The listing builds one solid part. Answer for the finished solid, in the listing's coordinates (mm). Coordinates: 2 decimals unless noted, no trailing zeros. Loops run counter-clockwise (first coordinate to the right, second up) from the corner with the lowest first, then second, coordinate; pieces in that order, holes last. Notation, with made-up numbers: (-15.5, 62) - (4.5, 62) arc R21 cw to (4.5, 97) - close; hole circle Ø9 at (39, -11). An arc over 180 degrees is marked (long way). Return JSON: item names as keys, results as strings. Group by question number.
1. Section B-B (z = 1.5) is taken. State how many separate pieces and enclosed holes the cut face has, and give its area (3 significant figures).
2. Each of these flat-tipped pins is pushed along its axis until it touches: P1, Ø0.8, axis at x = 399, z = 1.5, coming from the -Y side; P2, Ø0.6, axis at y = 21, z = 1, coming from the -X side. Where does it stop, or does it pass through?
3. Find the intervals of material crossed by line 1 along X through (y, z) = (32, 0.55); line 2 along Y through (x, z) = (221.5, 1.5); line 3 along Y through (x, z) = (230, 0.5), in increasing order.
4. Section A-A (x = 232) is taken. Write down the section's boundary in (y, z).
5. Section C-C (x = 328.5) is taken. Write down the section's boundary in (y, z).
```python
from build123d import *

# Parameters (mm, degrees)
SKETCH_2_W      = 1.5
SKETCH_2_H      = 6
EXTRUDE_2_DEPTH = 2


with BuildPart() as part:
    # 草图2 → 凸台-拉伸2 (new body)
    with BuildSketch(Plane.XY):
        Polygon((8.053783248, 22.194978349), (6.553783248, 22.194978349), (6.553783248, 28.194978349), (8.053783248, 28.194978349), (8.053783248, 34.194978349), (533.429113931, 35.353824286), (533.429113931, 5.627058882), (8.053783248, 16.095153128), align=None)
        with Locations((128.889742021, 24.455033291)):
            Rectangle(SKETCH_2_W, SKETCH_2_H, mode=Mode.SUBTRACT)
        with Locations((258.982626832, 23.318434437)):
            Rectangle(SKETCH_2_W, SKETCH_2_H, mode=Mode.SUBTRACT)
        with Locations((399.123508139, 22.161638966)):
            Rectangle(SKETCH_2_W, SKETCH_2_H, mode=Mode.SUBTRACT)
        with BuildLine():
            Line((14.053783248, 26.212604877), (14.053783248, 23.93734113))
            ThreePointArc((14.053783248, 23.93734113), (14.625552855, 22.537284723), (16.013941191, 21.937738017))
            Line((16.013941191, 21.937738017), (46.013941191, 21.339988544))
            ThreePointArc((46.013941191, 21.339988544), (47.453839655, 21.911361263), (48.053783248, 23.339591657))
            Line((48.053783248, 23.339591657), (48.053783248, 26.278777337))
            ThreePointArc((48.053783248, 26.278777337), (47.466436254, 27.694549736), (46.049371762, 28.278772471))
            Line((46.049371762, 28.278772471), (16.049371762, 28.212600011))
            ThreePointArc((16.049371762, 28.212600011), (14.638010849, 27.625257882), (14.053783248, 26.212604877))
        make_face(mode=Mode.SUBTRACT)
        with BuildLine():
            Line((52.053783248, 26.362790255), (52.053783248, 23.180191797))
            ThreePointArc((52.053783248, 23.180191797), (52.625552855, 21.78013539), (54.013941191, 21.180588684))
            Line((54.013941191, 21.180588684), (82.099899964, 20.620976448))
            ThreePointArc((82.099899964, 20.620976448), (83.539798428, 21.192349168), (84.139742021, 22.620579561))
            Line((84.139742021, 22.620579561), (84.139742021, 26.362790255))
            ThreePointArc((84.139742021, 26.362790255), (83.553955584, 27.777003817), (82.139742021, 28.362790255))
            Line((82.139742021, 28.362790255), (54.053783248, 28.362790255))
            ThreePointArc((54.053783248, 28.362790255), (52.639569686, 27.777003817), (52.053783248, 26.362790255))
        make_face(mode=Mode.SUBTRACT)
        with BuildLine():
            Line((88.139742021, 26.376019882), (88.139742021, 22.461179702))
            ThreePointArc((88.139742021, 22.461179702), (88.711511628, 21.061123295), (90.099899964, 20.461576589))
            Line((90.099899964, 20.461576589), (120.099899964, 19.863827115))
            ThreePointArc((120.099899964, 19.863827115), (121.539798428, 20.435199835), (122.139742021, 21.863430228))
            Line((122.139742021, 21.863430228), (122.139742021, 26.442192342))
            ThreePointArc((122.139742021, 26.442192342), (121.552395026, 27.857964741), (120.135330535, 28.442187476))
            Line((120.135330535, 28.442187476), (90.135330535, 28.376015016))
            ThreePointArc((90.135330535, 28.376015016), (88.723969622, 27.788672887), (88.139742021, 26.376019882))
        make_face(mode=Mode.SUBTRACT)
        with BuildLine():
            Line((135.639742021, 26.480792944), (135.639742021, 21.514743035))
            ThreePointArc((135.639742021, 21.514743035), (136.211511628, 20.114686628), (137.599899964, 19.515139922))
            Line((137.599899964, 19.515139922), (170.499899964, 18.859607999))
            ThreePointArc((170.499899964, 18.859607999), (171.939798428, 19.430980719), (172.539742021, 20.859211112))
            Line((172.539742021, 20.859211112), (172.539742021, 26.553362075))
            ThreePointArc((172.539742021, 26.553362075), (171.952395026, 27.969134474), (170.535330535, 28.553357209))
            Line((170.535330535, 28.553357209), (137.635330535, 28.480788078))
            ThreePointArc((137.635330535, 28.480788078), (136.223969622, 27.893445949), (135.639742021, 26.480792944))
        make_face(mode=Mode.SUBTRACT)
        with BuildLine():
            Line((176.539742021, 26.571008064), (176.539742021, 20.699811253))
            ThreePointArc((176.539742021, 20.699811253), (177.111511628, 19.299754846), (178.499899964, 18.70020814))
            Line((178.499899964, 18.70020814), (209.292784775, 18.08666045))
            ThreePointArc((209.292784775, 18.08666045), (210.732683239, 18.65803317), (211.332626832, 20.086263563))
            Line((211.332626832, 20.086263563), (211.332626832, 26.638929429))
            ThreePointArc((211.332626832, 26.638929429), (210.745279837, 28.054701828), (209.328215345, 28.638924564))
            Line((209.328215345, 28.638924564), (178.535330535, 28.571003199))
            ThreePointArc((178.535330535, 28.571003199), (177.123969622, 27.983661069), (176.539742021, 26.571008064))
        make_face(mode=Mode.SUBTRACT)
        with BuildLine():
            Line((215.332626832, 26.733560912), (215.332626832, 19.926863704))
            ThreePointArc((215.332626832, 19.926863704), (215.904396438, 18.526807297), (217.292784775, 17.92726059))
            Line((217.292784775, 17.92726059), (250.192784775, 17.271728668))
            ThreePointArc((250.192784775, 17.271728668), (251.632683239, 17.843101387), (252.232626832, 19.271331781))
            Line((252.232626832, 19.271331781), (252.232626832, 26.733560912))
            ThreePointArc((252.232626832, 26.733560912), (251.646840394, 28.147774475), (250.232626832, 28.733560912))
            Line((250.232626832, 28.733560912), (217.332626832, 28.733560912))
            ThreePointArc((217.332626832, 28.733560912), (215.918413269, 28.147774475), (215.332626832, 26.733560912))
        make_face(mode=Mode.SUBTRACT)
        with BuildLine():
            Line((265.732626832, 26.767745151), (265.732626832, 18.922644588))
            ThreePointArc((265.732626832, 18.922644588), (266.304396438, 17.522588181), (267.692784775, 16.923041475))
            Line((267.692784775, 16.923041475), (303.692784775, 16.205742106))
            ThreePointArc((303.692784775, 16.205742106), (305.132683239, 16.777114826), (305.732626832, 18.20534522))
            Line((305.732626832, 18.20534522), (305.732626832, 26.847152103))
            ThreePointArc((305.732626832, 26.847152103), (305.145279837, 28.262924503), (303.728215345, 28.847147238))
            Line((303.728215345, 28.847147238), (267.728215345, 28.767740286))
            ThreePointArc((267.728215345, 28.767740286), (266.316854432, 28.180398157), (265.732626832, 26.767745151))
        make_face(mode=Mode.SUBTRACT)
        with BuildLine():
            Line((309.732626832, 26.864798093), (309.732626832, 18.04594536))
            ThreePointArc((309.732626832, 18.04594536), (310.304396438, 16.645888953), (311.692784775, 16.046342247))
            Line((311.692784775, 16.046342247), (346.333666082, 15.356123294))
            ThreePointArc((346.333666082, 15.356123294), (347.773564547, 15.927496014), (348.373508139, 17.355726408))
            Line((348.373508139, 17.355726408), (348.373508139, 26.941207171))
            ThreePointArc((348.373508139, 26.941207171), (347.786161145, 28.35697957), (346.369096653, 28.941202305))
            Line((346.369096653, 28.941202305), (311.728215345, 28.864793227))
            ThreePointArc((311.728215345, 28.864793227), (310.316854432, 28.277451098), (309.732626832, 26.864798093))
        make_face(mode=Mode.SUBTRACT)
        with BuildLine():
            Line((352.373508139, 26.95885316), (352.373508139, 17.196326548))
            ThreePointArc((352.373508139, 17.196326548), (352.945277746, 15.796270141), (354.333666082, 15.196723435))
            Line((354.333666082, 15.196723435), (390.333666082, 14.479424066))
            ThreePointArc((390.333666082, 14.479424066), (391.773564547, 15.050796786), (392.373508139, 16.47902718))
            Line((392.373508139, 16.47902718), (392.373508139, 27.038260112))
            ThreePointArc((392.373508139, 27.038260112), (391.786161145, 28.454032511), (390.369096653, 29.038255247))
            Line((390.369096653, 29.038255247), (354.369096653, 28.958848295))
            ThreePointArc((354.369096653, 28.958848295), (352.95773574, 28.371506165), (352.373508139, 26.95885316))
        make_face(mode=Mode.SUBTRACT)
        with BuildLine():
            Line((405.873508139, 27.160684029), (405.873508139, 16.130339987))
            ThreePointArc((405.873508139, 16.130339987), (406.445277746, 14.73028358), (407.833666082, 14.130736874))
            Line((407.833666082, 14.130736874), (443.833666082, 13.413437505))
            ThreePointArc((443.833666082, 13.413437505), (445.273564547, 13.984810225), (445.873508139, 15.413040618))
            Line((445.873508139, 15.413040618), (445.873508139, 27.160684029))
            ThreePointArc((445.873508139, 27.160684029), (445.287721702, 28.574897591), (443.873508139, 29.160684029))
            Line((443.873508139, 29.160684029), (407.873508139, 29.160684029))
            ThreePointArc((407.873508139, 29.160684029), (406.459294577, 28.574897591), (405.873508139, 27.160684029))
        make_face(mode=Mode.SUBTRACT)
        with BuildLine():
            Line((449.873508139, 27.247933753), (449.873508139, 15.253640759))
            ThreePointArc((449.873508139, 15.253640759), (450.445277746, 13.853584352), (451.833666082, 13.254037646))
            Line((451.833666082, 13.254037646), (483.389271874, 12.625292754))
            ThreePointArc((483.389271874, 12.625292754), (484.829170338, 13.196665474), (485.429113931, 14.624895867))
            Line((485.429113931, 14.624895867), (485.429113931, 27.247933753))
            ThreePointArc((485.429113931, 27.247933753), (484.843327493, 28.662147316), (483.429113931, 29.247933753))
            Line((483.429113931, 29.247933753), (451.873508139, 29.247933753))
            ThreePointArc((451.873508139, 29.247933753), (450.459294577, 28.662147316), (449.873508139, 27.247933753))
        make_face(mode=Mode.SUBTRACT)
        with BuildLine():
            Line((489.429113931, 27.340575198), (489.429113931, 14.465496007))
            ThreePointArc((489.429113931, 14.465496007), (490.000883538, 13.0654396), (491.389271874, 12.465892894))
            Line((491.389271874, 12.465892894), (525.389271874, 11.788443491))
            ThreePointArc((525.389271874, 11.788443491), (526.829170338, 12.35981621), (527.429113931, 13.788046604))
            Line((527.429113931, 13.788046604), (527.429113931, 27.340575198))
            ThreePointArc((527.429113931, 27.340575198), (526.843327493, 28.75478876), (525.429113931, 29.340575198))
            Line((525.429113931, 29.340575198), (491.429113931, 29.340575198))
            ThreePointArc((491.429113931, 29.340575198), (490.014900369, 28.75478876), (489.429113931, 27.340575198))
        make_face(mode=Mode.SUBTRACT)
    extrude(amount=EXTRUDE_2_DEPTH)


solid = part.part
```
The answers:
{
 "1": {"separate pieces": "1", "enclosed holes": "15", "area": "7,320 mm2"},
 "2": {"P1": "stops at y = 8.3", "P2": "stops at x = 8.05"},
 "3": {"line 1": "x = 8.05 to 533.43", "line 2": "y = 11.84 to 17.84, 28.73 to 34.67", "line 3": "y = 11.67 to 17.67, 28.73 to 34.68"},
 "4": {"outline": "(11.63, 0) - (17.63, 0) - (17.63, 2) - (11.63, 2) - close; (28.73, 0) - (34.69, 0) - (34.69, 2) - (28.73, 2) - close"},
 "5": {"outline": "(9.71, 0) - (15.71, 0) - (15.71, 2) - (9.71, 2) - close; (28.9, 0) - (34.9, 0) - (34.9, 2) - (28.9, 2) - close"}
}
